Check sheet for the modelled part. Datum: model origin and axes. Units: mm. A direction names the side the tool comes from. Give positions to 0.01 mm unless a question says otherwise; leave off trailing zeros. Order: outer loops, then holes, each group sorted by start corner. A loop starts at its lowest first (then second) coordinate and runs counter-clockwise, first axis right, second up.
from build123d import *

# Parameters (mm, degrees)
BOSS_EXTRUDE1_DEPTH       = 30
M4X0_7_TAPPED_HOLE1_D     = 3.3
M4X0_7_TAPPED_HOLE1_DEPTH = 10.1
M4X0_7_TAPPED_HOLE1_TIP   = 0.991420021
SKETCH4_R                 = 3.556
BOSS_EXTRUDE2_DEPTH       = 5
FILLET1_R                 = 5


with BuildPart() as part:
    # Sketch1 → Boss-Extrude1 (new body)
    with BuildSketch(Plane(origin=(0, 0, 0), x_dir=(1, 0, 0), z_dir=(0, 1, 0))):
        with BuildLine():
            Line((-10, -7), (10, -7))
            ThreePointArc((10, -7), (17, 0), (10, 7))
            Line((10, 7), (-10, 7))
            ThreePointArc((-10, 7), (-17, 0), (-10, -7))
        make_face()
    extrude(amount=BOSS_EXTRUDE1_DEPTH)

    # M4x0.7 Tapped Hole1
    with Locations(Plane(origin=(0, 30, 0), x_dir=(1, 0, 0), z_dir=(0, 1, 0))):
        with Locations((-10, 0), (10, 0)):
            Hole(M4X0_7_TAPPED_HOLE1_D / 2, depth=M4X0_7_TAPPED_HOLE1_DEPTH)
            with Locations((0, 0, -(M4X0_7_TAPPED_HOLE1_DEPTH + M4X0_7_TAPPED_HOLE1_TIP / 2))):  # 118° drill point
                Cone(0, M4X0_7_TAPPED_HOLE1_D / 2, M4X0_7_TAPPED_HOLE1_TIP, mode=Mode.SUBTRACT)

    # Sketch4 → Boss-Extrude2 (add)
    with BuildSketch(Plane.XZ):
        with BuildLine():
            Line((6, 12.7), (6, -12.7))
            ThreePointArc((6, -12.7), (0, -18.7), (-6, -12.7))
            Line((-6, -12.7), (-6, 12.7))
            ThreePointArc((-6, 12.7), (0, 18.7), (6, 12.7))
        make_face()
        with Locations(Location((0, 12.7, 0), (0, 0, 270))):
            Circle(SKETCH4_R, mode=Mode.SUBTRACT)
        with Locations(Location((0, -12.7, 0), (0, 0, 270))):
            Circle(SKETCH4_R, mode=Mode.SUBTRACT)
    extrude(amount=-BOSS_EXTRUDE2_DEPTH)

    # Fillet1
    # the kernel refuses this fillet: 5 mm, written as the material it adds along each edge
    with BuildSketch(Plane(origin=(-6, 5, 7), x_dir=(-0.9999858901973535, 0, -0.0053121941047544466), z_dir=(0, -1, 0)), Plane(origin=(-6, 0, -7), x_dir=(-0.9999858901973535, 0, 0.005312194104754061), z_dir=(0, 1, 0)), Plane(origin=(6, 5, -7), x_dir=(0.9999858901973535, 0, 0.005312194104753284), z_dir=(0, -1, 0)), Plane(origin=(6, 0, 7), x_dir=(0.9999858901973535, 0, -0.0053121941047534794), z_dir=(0, 1, 0))) as fillet1_piece_1:
        with BuildLine():
            CenterArc((4.973590207, -4.984751754), FILLET1_R, 94.475824114, 85.219808153)
            Line((-0.026339243, -4.958190783), (-0.526332189, -4.955534686))
            Line((-0.526332189, -4.955534686), (-0.499992945, 0.002656097))
            Line((-0.499992945, 0.002656097), (0.002656097, 0.499992945))
            ThreePointArc((0.002656097, 0.499992945), (4.002599658, 0.478744169), (4.544378784, 0.498475175))
            Line((4.544378784, 0.498475175), (4.583398004, 0))
        make_face()
    extrude(amount=5)


solid = part.part
1) Section check B-B, the plane z = -14.5. Record the cut outline in (x, y), then the cut area to 3 significant figures.
Recorded:
outline: (-5.72, 0) - (-3.07, 0) - (-3.07, 5) - (-5.72, 5) - close; (3.07, 0) - (5.72, 0) - (5.72, 5) - (3.07, 5) - close
area: 26.6 mm2
2) Set-up check for faces 5 (the face through (-0.2, 5, 8.8)), 6 (the face through (-0.2, 5, -8.8)), 7 (the face through (8.476, 24.879, 0.632)): record each of +Z, -Z, +X, -X, +Y, -Y from which the full face is reachable in a straight line by a thin tool's end or side.
Recorded:
face 5: +Z, +X, -X, +Y
face 6: -Z, +X, -X, +Y
face 7: +Y
3) Section check D-D, the plane y = 11.25. Record the cut outline in (x, z).
Recorded:
outline: (-10, -7) - (10, -7) arc R7 ccw to (10, 7) - (-10, 7) arc R7 ccw to start
4) Depth check by flat-ended pin: pin 1 Ø16 at (x, y) = (1, 23) entering from +Z; pin 2 Ø3.5 at (x, z) = (-3.5, -10.5) entering from +Y; pin 3 Ø6 at (x, y) = (3, 21) entering from -Z; pin 4 Ø6.5 at (x, z) = (0, 12.7) entering from -Y. Enter the tip coordinate at first touch or a pass-through.
Recorded:
pin 1: stops at z = 7
pin 2: stops at y = 5
pin 3: stops at z = -7
pin 4: passes through
5) Draft check along X on faces 1 (the face through (0, 0, 0)), 2 (the face through (0.1, 2.5, -18.7)), 3 (the face through (-1.362, 2.465, -15.985)), 4 (the face through (-9.7, 19.1, 0.1)). Enter one of: +X half, -X half, draft (parallel to the pull), parting line (faces both ways), or undercut.
Recorded:
face 1: draft
face 2: parting line
face 3: undercut
face 4: undercut
6) Material ranges on L1, parallel to Z at x = 10, y = 25.75; L2, parallel to X at y = 3.1, z = -12.7; L3, parallel to Y at x = -6, z = -9.5, recorded low to high.
Recorded:
L1: z = -7 to -1.65, 1.65 to 7
L2: x = -6 to -3.56, 3.56 to 6
L3: y = 0 to 5
7) Section check A-A, the plane x = 0. Record the cut outline in (y, z).
Recorded:
outline: (0, -18.7) - (5, -18.7) - (5, -16.26) - (0, -16.26) - close; (0, -9.14) - (5, -9.14) - (5, -7) - (30, -7) - (30, 7) - (5, 7) - (5, 9.14) - (0, 9.14) - close; (0, 16.26) - (5, 16.26) - (5, 18.7) - (0, 18.7) - close
8) Section check C-C, the plane y = 21. Record the cut outline in (x, z).
Recorded:
outline: (-10, -7) - (10, -7) arc R7 ccw to (10, 7) - (-10, 7) arc R7 ccw to start; hole circle Ø3.3 at (-10, 0); hole circle Ø3.3 at (10, 0)
